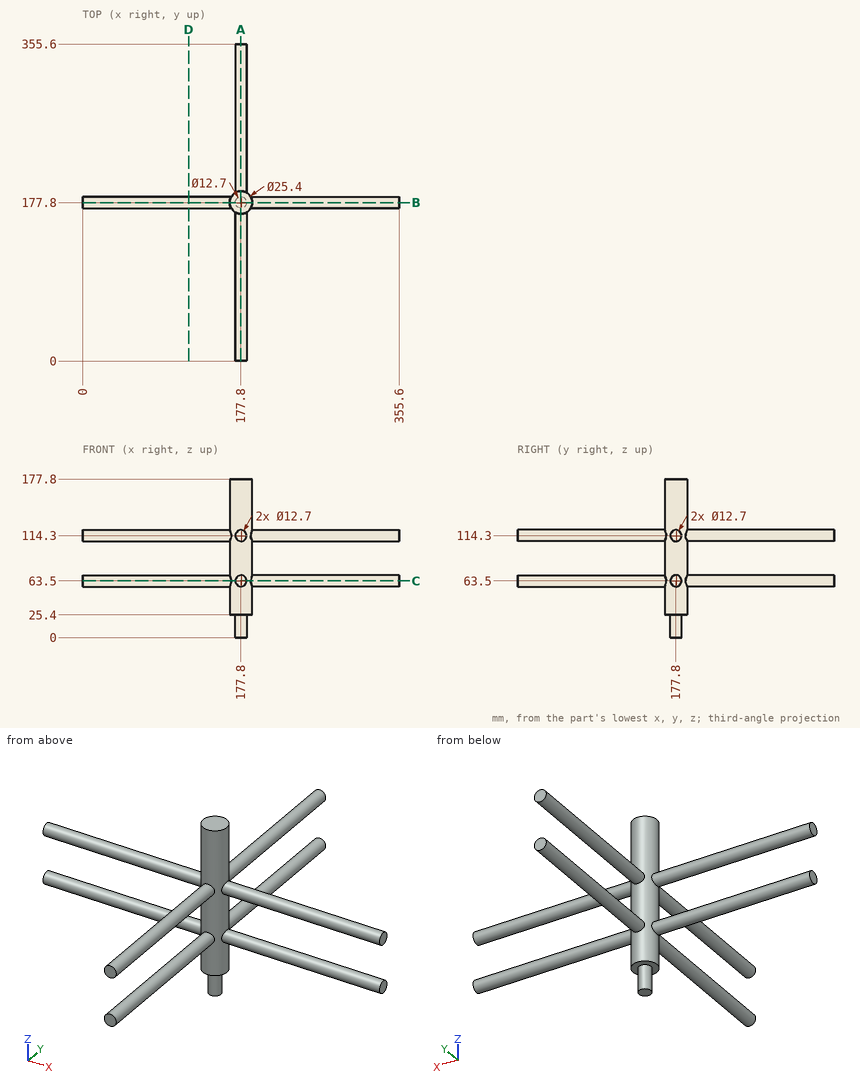
Verification items for this drawing (mm, ordinates from the low corner). Coordinates: 2 decimals unless noted, no trailing zeros. Write each loop counter-clockwise with the first axis right and the second up, starting at its lowest first coordinate (ties: lowest second). Pieces come first, ordered by that corner, then holes. Notation, with made-up numbers: (6.25, 89.25) -> (48.25, 89.25) arc R22 cw to (48.25, 108.25) -> close; hole circle Ø1 at (-25.75, -0.5). An arc over 180 degrees is marked (long way). Use CSV: the item, a comma, the result in double quotes. Start each with the question number.
Item 1: Cross-section at C-C, the plane z = 63.5. Record the cut outline in (x, y).
Item 2: Thickness scan on line 1 (X direction, y = 105.5, z = 114); line 2 (Y direction, x = 189, z = 160); line 3 (Y direction, x = 97.5, z = 111). Record the ranges inside material, lowest first.
Item 3: Cross-section at A-A, the plane x = 177.8. Record the cut outline in (y, z), plus the area to 3 significant figures.
Item 4: Depth check by flat-ended pin: pin 1 Ø4 at (y, z) = (174.5, 148.5) entering from -X; pin 2 Ø6 at (x, z) = (169.5, 55.5) entering from +Y. Enter the tip coordinate at first touch or a pass-through.
Item 5: Cross-section at D-D, the plane x = 119. Record the cut outline in (y, z).
Answers:
1,outline,"(0, 171.45) -> (166.8, 171.45) arc R12.7 ccw to (171.45, 166.8) -> (171.45, 0) -> (184.15, 0) -> (184.15, 166.8) arc R12.7 ccw to (188.8, 171.45) -> (355.6, 171.45) -> (355.6, 184.15) -> (188.8, 184.15) arc R12.7 ccw to (184.15, 188.8) -> (184.15, 355.6) -> (171.45, 355.6) -> (171.45, 188.8) arc R12.7 ccw to (166.8, 184.15) -> (0, 184.15) -> close"
2,line 1,"171.46 to 184.14"
2,line 2,"171.81 to 183.79"
2,line 3,"172.37 to 183.23"
3,outline,"(0, 57.15) -> (165.1, 57.15) -> (165.1, 25.4) -> (171.45, 25.4) -> (171.45, 0) -> (184.15, 0) -> (184.15, 25.4) -> (190.5, 25.4) -> (190.5, 57.15) -> (355.6, 57.15) -> (355.6, 69.85) -> (190.5, 69.85) -> (190.5, 107.95) -> (355.6, 107.95) -> (355.6, 120.65) -> (190.5, 120.65) -> (190.5, 177.8) -> (165.1, 177.8) -> (165.1, 120.65) -> (0, 120.65) -> (0, 107.95) -> (165.1, 107.95) -> (165.1, 69.85) -> (0, 69.85) -> close"
3,area,"12,600 mm^2"
4,pin 1,"x = 165.17"
4,pin 2,"y = 189.34"
5,outline,"circle Ø12.7 at (177.8, 63.5); circle Ø12.7 at (177.8, 114.3)"
